```python
from build123d import *

# Parameters (mm, degrees)
SKETCH1_W                      = 12
SKETCH1_H                      = 8
BOSS_EXTRUDE1_DEPTH            = 700
CBORE_FOR_M3_SHCS1_D           = 3.4
CBORE_FOR_M3_SHCS1_CBORE_D     = 6.5
CBORE_FOR_M3_SHCS1_CBORE_DEPTH = 3


with BuildPart() as part:
    # Sketch1 → Boss-Extrude1 (new body)
    with BuildSketch(Plane.XY):
        with Locations((6, 4)):
            Rectangle(SKETCH1_W, SKETCH1_H)
    extrude(amount=BOSS_EXTRUDE1_DEPTH)

    # CBORE for M3 SHCS1 (through all)
    with Locations(Plane(origin=(0, 8, 0), x_dir=(1, 0, 0), z_dir=(0, 1, 0))):
        with Locations((6, -690), (6, -665), (6, -640), (6, -615), (6, -590), (6, -565), (6, -540), (6, -515), (6, -490), (6, -465), (6, -440), (6, -415), (6, -390), (6, -365), (6, -340), (6, -315), (6, -290), (6, -265), (6, -240), (6, -215), (6, -190), (6, -165), (6, -140), (6, -115), (6, -90), (6, -65), (6, -40), (6, -15)):
            CounterBoreHole(CBORE_FOR_M3_SHCS1_D / 2, CBORE_FOR_M3_SHCS1_CBORE_D / 2, CBORE_FOR_M3_SHCS1_CBORE_DEPTH)


solid = part.part
```
Input: part model. Units: mm. Frame: model coordinates. Round coordinates to 2 decimals unless told otherwise and drop trailing zeros. Use one line per item in the form item = value. Start each with the question number.
Item 1: Contact query for a flat-ended pin moving along its axis: pin 1 Ø4 at (x, z) = (6, 615) entering from +Y. Output: stop coordinate, or through.
Item 2: Section query A-A on y = 1.25. Count the separate pieces of the cut face and the enclosed holes in it, then the cut area to 3 significant figures.
Item 3: Material intervals for L1, parallel to X at y = 6.45, z = 490; L2, parallel to X at y = 2.4, z = 165; L3, parallel to Y at x = 3.5, z = 365.5, sorted ascending. Write a range as from..to.
Ans:
q1.pin_1 = 5
q2.separate_pieces = 1
q2.enclosed_holes = 28
q2.area = 8,150 mm^2
q3.L1 = 0..2.75, 9.25..12
q3.L2 = 0..4.3, 7.7..12
q3.L3 = 0..5
